Answer from the drawing. Dimensions are ordinates in mm from the lowest x, y and z of the part. A direction names the side the tool comes from. Coordinates: 2 decimals unless noted, no trailing zeros. Order: outer loops, then holes, each group sorted by start corner. A loop starts at its lowest first (then second) coordinate and runs counter-clockwise, first axis right, second up. Notation, with made-up numbers: (28, 7.25) - (61, 7.25) arc R19 ccw to (61, 20.25) - close; hole circle Ø11 at (-30, 11). An arc over 180 degrees is marked (long way). One line per item, written item: value. Start each with the question number.
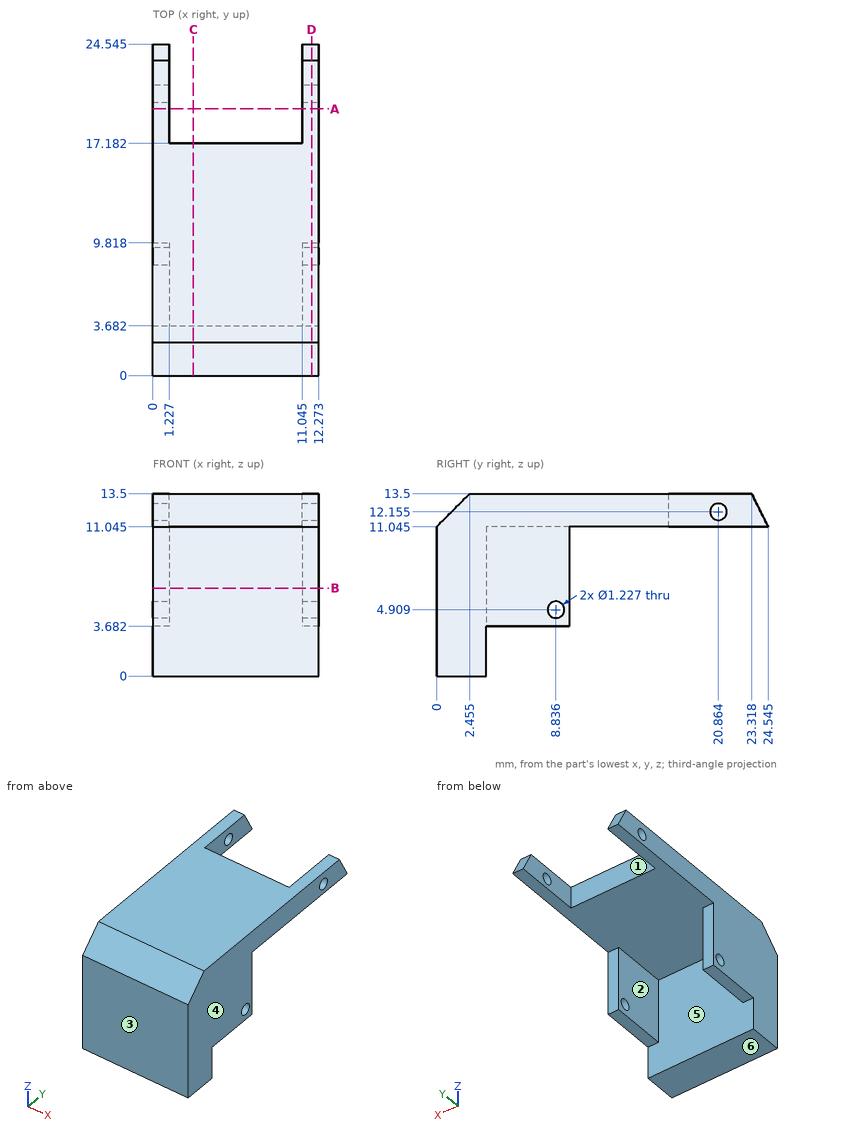
(1) The part is cut by section D-D on x = 11.75. Count the separate pieces of the cut face and the enclosed holes in it, plus the area to 3 significant figures.
(2) The part is cut by section A-A on y = 19.75. Determine the outline of the cut face in (x, z) (1 decimal).
(3) The part is cut by section C-C on x = 3. Determine the outline of the cut face in (y, z) (1 decimal).
(4) For the marked faces 1, 2 and 3, determine the directions among +Z, -Z, +X, -X, +Y, -Y from which every point of the face is accessible in a straight line to the end or side of a thin tool.
(5) Flat-ended cylindrical pins translate along their axes: pin 1 Ø0.6 at (x, y) = (0.5, 7) entering from -Z; pin 2 Ø6 at (y, z) = (15.5, 6) entering from -X; pin 3 Ø4 at (x, y) = (2.5, 17.5) entering from +Z; pin 4 Ø0.6 at (x, z) = (0.5, 8.5) entering from +Y. Find the tip coordinate at first contact, or state that the pin passes through.
(6) The part is cut by section B-B on z = 6.5. Determine the outline of the cut face in (x, y) (1 decimal).
(7) Consider probe 1 along X at (y, z) = (8.75, 6.5) (1 decimal); probe 2 along Y at (x, z) = (9.5, 4.5); probe 3 along Z at (x, y) = (5.75, 11) (1 decimal). Determine where each line is inside the solid, lowest interval first.
(8) For a pull along X with two mould halves and no side action, classify the marked faces 4, 5 and 6 as pulls with the +X half, pulls with the -X half, needs draft (parallel to the pull), parting line crosses it, or undercut.
Completed:
1. separate pieces: 1
1. enclosed holes: 2
1. area: 139 mm2
2. outline: (0, 11) - (1.2, 11) - (1.2, 13.5) - (0, 13.5) - close; (11, 11) - (12.3, 11) - (12.3, 13.5) - (11, 13.5) - close
3. outline: (0, 0) - (3.7, 0) - (3.7, 11) - (17.2, 11) - (17.2, 13.5) - (2.5, 13.5) - (0, 11) - close
4. face 1: +Z, -Z, +Y
4. face 2: -Z, +Y
4. face 3: +Z, -Z, +X, -X, -Y
5. pin 1: stops at z = 3.68
5. pin 2: passes through
5. pin 3: stops at z = 13.5
5. pin 4: stops at y = 9.82
6. outline: (0, 0) - (12.3, 0) - (12.3, 9.8) - (11, 9.8) - (11, 3.7) - (1.2, 3.7) - (1.2, 9.8) - (0, 9.8) - close
7. probe 1: x = 0 to 1.2, 11 to 12.3
7. probe 2: y = 0 to 3.68
7. probe 3: z = 11 to 13.5
8. face 4: pulls with the +X half
8. face 5: undercut
8. face 6: needs draft
